from build123d import *

# Parameters (mm, degrees)
EXTRUDE_START       = -10
SKETCH_1_R          = 20
SKETCH_1_R_2        = 11
EXTRUDE_1_DEPTH     = 50
SKETCH_2_R          = 39
SKETCH_2_R_2        = 10.9
EXTRUDE_2_DEPTH     = 10
CHAMFER_1_SIZE      = 4
SKETCH_3_R          = 35
SKETCH_3_R_2        = 17
EXTRUDE_3_DEPTH     = 7
CHAMFER_2_SIZE      = 3
SKETCH_4_R          = 3.000000009
CUT_EXTRUDE_1_DEPTH = 64.765194268
CUT_EXTRUDE_4_REACH = 83.498
SKETCH_5_R          = 3


with BuildPart() as part:
    # Эскиз1 → Вытянуть1 (new body)
    with BuildSketch(Plane(origin=(0, 0, 0), x_dir=(1, 0, 0), z_dir=(0, 1, 0)).offset(EXTRUDE_START)):
        with Locations(Location((0, 0, 0), (0, 0, 270))):
            Circle(SKETCH_1_R)
        with Locations(Location((0, 0, 0), (0, 0, 270))):
            Circle(SKETCH_1_R_2, mode=Mode.SUBTRACT)
    extrude(amount=EXTRUDE_1_DEPTH)

    # Эскиз2 → Вытянуть2 (add)
    with BuildSketch(Plane(origin=(0, 40, 0), x_dir=(1, 0, 0), z_dir=(0, 1, 0))):
        with Locations(Location((0, 0, 0), (0, 0, 270))):
            Circle(SKETCH_2_R)
        with Locations(Location((0, 0, 0), (0, 0, 270))):
            Circle(SKETCH_2_R_2, mode=Mode.SUBTRACT)
    extrude(amount=EXTRUDE_2_DEPTH)

    # Фаска1
    chamfer_1_edges = [part.edges().sort_by_distance(p)[0] for p in [
        (0, 40, -20),
    ]]
    chamfer(chamfer_1_edges, length=CHAMFER_1_SIZE)

    # Эскиз3 → Вытянуть3 (add)
    with BuildSketch(Plane.XZ.offset(-15)):
        with Locations(Location((0, 0, 0), (0, 0, 270))):
            Circle(SKETCH_3_R)
        Circle(SKETCH_3_R_2, mode=Mode.SUBTRACT)
    extrude(amount=-EXTRUDE_3_DEPTH)

    # Фаска2
    chamfer_2_edges = [part.edges().sort_by_distance(p)[0] for p in [
        (0, 22, -20),
    ]]
    chamfer(chamfer_2_edges, length=CHAMFER_2_SIZE)

    # Эскиз4 → Вырез-Вытянуть1 (cut, through all)
    with BuildSketch(Plane(origin=(0, 22, 0), x_dir=(1, 0, 0), z_dir=(0, 1, 0))):
        with Locations(Location((-13.413764566, 24.758384407, 0), (0, 0, 270))):
            Circle(SKETCH_4_R)
        with Locations(Location((14.742626006, 23.99086611, 0), (0, 0, 270))):
            Circle(SKETCH_4_R)
        with Locations(Location((28.156130949, -0.777042552, 0), (0, 0, 270))):
            Circle(SKETCH_4_R)
        with Locations(Location((13.41324532, -24.777432917, 0), (0, 0, 270))):
            Circle(SKETCH_4_R)
        with Locations(Location((-14.743145251, -24.009914621, 0), (0, 0, 270))):
            Circle(SKETCH_4_R)
        with Locations(Location((-28.156650194, 0.757994041, 0), (0, 0, 270))):
            Circle(SKETCH_4_R)
    extrude(amount=-CUT_EXTRUDE_1_DEPTH, mode=Mode.SUBTRACT)

    # Эскиз5 → Вытянуть4 (cut, up to next)
    with BuildSketch(Plane(origin=(0, 50, 0), x_dir=(1, 0, 0), z_dir=(0, 1, 0)), mode=Mode.PRIVATE) as cut_extrude_4_sk1:
        with Locations(Location((0, 31, 0), (0, 0, 270))):
            Circle(SKETCH_5_R)
    cut_extrude_4_tool1 = extrude(cut_extrude_4_sk1.sketch, amount=-CUT_EXTRUDE_4_REACH, mode=Mode.PRIVATE) & part.part
    # Эскиз5 → Вытянуть4 (cut, up to next)
    with BuildSketch(Plane(origin=(0, 50, 0), x_dir=(1, 0, 0), z_dir=(0, 1, 0)), mode=Mode.PRIVATE) as cut_extrude_4_sk2:
        with Locations(Location((26.846787517, 15.5, 0), (0, 0, 270))):
            Circle(SKETCH_5_R)
    cut_extrude_4_tool2 = extrude(cut_extrude_4_sk2.sketch, amount=-CUT_EXTRUDE_4_REACH, mode=Mode.PRIVATE) & part.part
    # Эскиз5 → Вытянуть4 (cut, up to next)
    with BuildSketch(Plane(origin=(0, 50, 0), x_dir=(1, 0, 0), z_dir=(0, 1, 0)), mode=Mode.PRIVATE) as cut_extrude_4_sk3:
        with Locations(Location((26.846787517, -15.5, 0), (0, 0, 270))):
            Circle(SKETCH_5_R)
    cut_extrude_4_tool3 = extrude(cut_extrude_4_sk3.sketch, amount=-CUT_EXTRUDE_4_REACH, mode=Mode.PRIVATE) & part.part
    # Эскиз5 → Вытянуть4 (cut, up to next)
    with BuildSketch(Plane(origin=(0, 50, 0), x_dir=(1, 0, 0), z_dir=(0, 1, 0)), mode=Mode.PRIVATE) as cut_extrude_4_sk4:
        with Locations(Location((0, -31, 0), (0, 0, 270))):
            Circle(SKETCH_5_R)
    cut_extrude_4_tool4 = extrude(cut_extrude_4_sk4.sketch, amount=-CUT_EXTRUDE_4_REACH, mode=Mode.PRIVATE) & part.part
    # Эскиз5 → Вытянуть4 (cut, up to next)
    with BuildSketch(Plane(origin=(0, 50, 0), x_dir=(1, 0, 0), z_dir=(0, 1, 0)), mode=Mode.PRIVATE) as cut_extrude_4_sk5:
        with Locations(Location((-26.846787517, -15.5, 0), (0, 0, 270))):
            Circle(SKETCH_5_R)
    cut_extrude_4_tool5 = extrude(cut_extrude_4_sk5.sketch, amount=-CUT_EXTRUDE_4_REACH, mode=Mode.PRIVATE) & part.part
    # Эскиз5 → Вытянуть4 (cut, up to next)
    with BuildSketch(Plane(origin=(0, 50, 0), x_dir=(1, 0, 0), z_dir=(0, 1, 0)), mode=Mode.PRIVATE) as cut_extrude_4_sk6:
        with Locations(Location((-26.846787517, 15.5, 0), (0, 0, 270))):
            Circle(SKETCH_5_R)
    cut_extrude_4_tool6 = extrude(cut_extrude_4_sk6.sketch, amount=-CUT_EXTRUDE_4_REACH, mode=Mode.PRIVATE) & part.part
    add(cut_extrude_4_tool1.solids().sort_by_distance((0, 50, -31))[0], mode=Mode.SUBTRACT)
    add(cut_extrude_4_tool2.solids().sort_by_distance((26.846788, 50, -15.5))[0], mode=Mode.SUBTRACT)
    add(cut_extrude_4_tool3.solids().sort_by_distance((26.846788, 50, 15.5))[0], mode=Mode.SUBTRACT)
    add(cut_extrude_4_tool4.solids().sort_by_distance((0, 50, 31))[0], mode=Mode.SUBTRACT)
    add(cut_extrude_4_tool5.solids().sort_by_distance((-26.846788, 50, 15.5))[0], mode=Mode.SUBTRACT)
    add(cut_extrude_4_tool6.solids().sort_by_distance((-26.846788, 50, -15.5))[0], mode=Mode.SUBTRACT)


solid = part.part
Input: part model. Units: mm. Frame: model coordinates. A direction names the side the tool comes from. Round coordinates to 2 decimals unless told otherwise and drop trailing zeros. Write each loop counter-clockwise with the first axis right and the second up, starting at its lowest first coordinate (ties: lowest second). Pieces come first, ordered by that corner, then holes.
1) Cut plane C-C (y = 12). Return the cut outline in (x, z), then the cut area to 3 significant figures.
2) Reachability of faces 1 (the cylindrical face through (23.92, 45.07, 14.85)), 2 (the cylindrical face through (-21, 18, 28)), 3 (the conical face through (-19.974, 24.854, -2.623)), 4 (the cylindrical face through (38.668, 44.93, -5.077)), 5 (the flat face through (-8, 50, 8)) from +Z, -Z, +X, -X, +Y, -Y: full face, straight path, thin tool, end or side. Return the list, or none.
3) Contact query for flat-ended pins moving along their axis: P1, Ø5.5, axis at x = -13.41, z = -24.76, coming from the -Y side; P2, Ø4, axis at y = 30.5, z = -14, coming from the +X side; P3, Ø10, axis at y = -3.5, z = 7, coming from the -X side; P4, Ø9.5, axis at x = 0, z = -31, coming from the +Y side. Output: stop coordinate, or through.
4) Ray query, L1, parallel to Y at x = -24, z = -6; L2, parallel to X at y = 43.25, z = -15.5; L3, parallel to Y at x = 19, z = -31.5. Return the intervals inside material, ascending.
5) Cut plane B-B (y = 44.5). Return the cut outline in (x, z), then the cut area to 3 significant figures.
6) Cut plane D-D (z = 0). Count the separate pieces of the cut face and the enclosed holes in it, then the cut area to 3 significant figures.
7) Cut plane A-A (z = -31). Return the cut outline in (x, y).
8) Draft query along Y for faces 6 (the flat face through (-9, -10, 9)), 7 (the flat face through (-7, 22, -23)), 8 (the cylindrical face through (-10.74, 14.65, -2.38)). Return one class per face: pulls with the +Y half, pulls with the -Y half, needs draft (parallel to the pull), parting line crosses it, or undercut.
Geometry says:
1. outline: circle Ø40 at (0, 0); hole circle Ø22 at (0, 0)
1. area: 877 mm2
2. face 1: +Y
2. face 2: -Y
2. face 3: none
2. face 4: +Y, -Y
2. face 5: +Z, -Z, +X, -X, +Y
3. P1: stops at y = 40
3. P2: stops at x = 16
3. P3: stops at x = -19.9
3. P4: stops at y = 50
4. L1: y = 15 to 22, 40 to 50
4. L2: x = -35.79 to -29.85, -23.85 to 23.85, 29.85 to 35.79
4. L3: y = 40 to 50
5. outline: circle Ø78 at (0, 0); hole circle Ø6 at (-26.85, -15.5); hole circle Ø6 at (-26.85, 15.5); hole circle Ø21.8 at (0, 0); hole circle Ø6 at (0, -31); hole circle Ø6 at (0, 31); hole circle Ø6 at (26.85, -15.5); hole circle Ø6 at (26.85, 15.5)
5. area: 4,240 mm2
6. separate pieces: 4
6. enclosed holes: 0
6. area: 1,620 mm2
7. outline: (-23.66, 40) - (-3, 40) - (-3, 50) - (-23.66, 50) - close; (-16.25, 15) - (16.25, 15) - (16.25, 22) - (-16.25, 22) - close; (3, 40) - (23.66, 40) - (23.66, 50) - (3, 50) - close
8. face 6: pulls with the -Y half
8. face 7: undercut
8. face 8: needs draft
